Autodesk Inventor part; units mm, degrees
ref_plane "YZ Plane" through (0, 0, 0) normal (1, 0, 0) x (0, 1, 0)
ref_plane "XZ Plane" through (0, 0, 0) normal (0, 1, 0) x (-1, 0, 0)
ref_plane "XY Plane" through (0, 0, 0) normal (0, 0, 1) x (1, 0, 0)
sketch "Sketch1" plane through (0, 0, 0) normal (0, 0, 1) x (1, 0, 0)
  line L0 (-46.5, 0) -> (-46.5, -19.95)
  line L1 (-46.5, -19.95) -> (-43.5, -19.95)
  arc A0 (-6.9796, -66.5) -> (-43.5, -29.9796) centre (-45, -68) ccw
  line L2 (-43.5, -19.95) -> (-43.5, -29.9796)
  line L3 (-3, 0) -> (-3, -54.5)
  line L4 (-3, -54.5) -> (0, -54.5)
  line L5 (-20, 0) -> (-20, 3)
  line L6 (-20, 3) -> (-30, 3)
  line L7 (-30, 3) -> (-30, 0)
  line L8 (-46.5, 0) -> (-30, 0)
  line L9 (-20, 0) -> (-3, 0)
  line L10 (-3, -69.5) -> (-3, -66.5)
  line L11 (-38.5, -20.7078) -> (-38.5, -7)
  line L12 (-36.5, -5) -> (-10, -5)
  line L13 (-8, -7) -> (-8, -35.0788)
  arc A1 (-11.4568, -36.4491) -> (-36.8538, -22.6763) centre (-45, -68) ccw
  arc A2 (-38.5, -20.7078) -> (-36.8538, -22.6763) centre (-36.5, -20.7078) ccw
  arc A3 (-36.5, -5) -> (-38.5, -7) centre (-36.5, -7) ccw
  arc A4 (-8, -7) -> (-10, -5) centre (-10, -7) ccw
  arc A5 (-11.4568, -36.4491) -> (-8, -35.0788) centre (-10, -35.0788) ccw
  line L14 (-3, -66.5) -> (-6.9796, -66.5)
  line L15 (-3, -69.5) -> (0, -69.5)
  line L16 (46.5, 0) -> (46.5, -19.95)
  line L17 (46.5, -19.95) -> (43.5, -19.95)
  arc A6 (43.5, -29.9796) -> (6.9796, -66.5) centre (45, -68) ccw
  line L18 (43.5, -19.95) -> (43.5, -29.9796)
  line L19 (3, 0) -> (3, -54.5)
  line L20 (3, -54.5) -> (0, -54.5)
  line L21 (20, 0) -> (20, 3)
  line L22 (20, 3) -> (30, 3)
  line L23 (30, 3) -> (30, 0)
  line L24 (46.5, 0) -> (30, 0)
  line L25 (20, 0) -> (3, 0)
  line L26 (3, -69.5) -> (3, -66.5)
  line L27 (38.5, -20.7078) -> (38.5, -7)
  line L28 (36.5, -5) -> (10, -5)
  line L29 (8, -7) -> (8, -35.0788)
  arc A7 (36.8538, -22.6763) -> (11.4568, -36.4491) centre (45, -68) ccw
  arc A8 (36.8538, -22.6763) -> (38.5, -20.7078) centre (36.5, -20.7078) ccw
  arc A9 (38.5, -7) -> (36.5, -5) centre (36.5, -7) ccw
  arc A10 (10, -5) -> (8, -7) centre (10, -7) ccw
  arc A11 (8, -35.0788) -> (11.4568, -36.4491) centre (10, -35.0788) ccw
  line L30 (3, -66.5) -> (6.9796, -66.5)
  line L31 (3, -69.5) -> (0, -69.5)
  point P0 (0, 0)
  point P1 (-8, -40.5846)
  point P2 (-38.5, -22.411)
  point P3 (8, -40.5846)
  point P4 (38.5, -22.411)
  dimension "d1" = 46.5
  dimension "d3" = 3
  dimension "d5" = 76.1
  dimension "d7" = 45
  dimension "d10" = 10
  dimension "d24" = 10
  dimension "d25" = 20
  dimension "d29" = 3
  dimension "d32" = 8
  dimension "d33" = 5
  dimension "d36" = 17
  dimension "d37" = 16.5
  dimension "d38" = 19.95
  dimension "d39" = 5
  dimension "d40" = 2
  dimension "d45" = 8
  dimension "d49" = 69.5
  dimension "d50" = 15
extrude "Extrusion4" add sketch "Sketch1" along normal blind 3
properties part number "OpenROV 2_2 Aft Ducting Brace"
Work out the finished part from the listing and answer in its coordinate system (mm). A direction names the side the tool comes from. Round coordinates to 2 decimals unless told otherwise and drop trailing zeros. Loops run counter-clockwise (first coordinate to the right, second up) from the corner with the lowest first, then second, coordinate; pieces in that order, holes last. Notation, with made-up numbers: M 38.5,14 L 44.5,14 A25 cw 44.5,45 Z; hole C 21,-18 d7. An arc over 180 degrees is marked long. Use CSV: the item, a comma, the result in double quotes.
Q1. Section D-D, the plane z = 1.55 is taken. State how many separate pieces and enclosed holes the cut face has, then the cut area to 3 significant figures.
Determined:
separate pieces,"1"
enclosed holes,"2"
area,"2,180 mm2"
Q2. The mould has two halves that part along Y. Classify faces 5 (the flat face through (43.5, -25, 1)), 6 (the cylindrical face through (-18.377, -40.815, 1.479)), 7 (the flat face through (-23, -5, 1)): pulls with the +Y half, pulls with the -Y half, needs draft (parallel to the pull), parting line crosses it, or undercut.
Determined:
face 5,"needs draft"
face 6,"pulls with the -Y half"
face 7,"undercut"
Q3. A tool of negligible diameter and unlimited length cuts with its end or side. For faces 1 (the flat face through (5, -66.5, 1)), 2 (the flat face through (12, 0, 1)), 3 (the cylindrical face through (8.57, -5.6, 1.48)), 4 (the flat face through (-5, -66.5, 1)), from which of +Z, -Z, +X, -X, +Y, -Y can it reach the whole face along a straight path? Write none if from no direction.
Determined:
face 1,"+Z, -Z, +X, -Y"
face 2,"+Z, -Z, +Y"
face 3,"+Z, -Z"
face 4,"+Z, -Z, -X, -Y"
Q4. Section A-A, the plane y = -8 is taken. Determine the outline of the cut face in (x, z).
Determined:
outline,"M -46.5,0 L -38.5,0 L -38.5,3 L -46.5,3 Z; M -8,0 L -3,0 L -3,3 L -8,3 Z; M 3,0 L 8,0 L 8,3 L 3,3 Z; M 38.5,0 L 46.5,0 L 46.5,3 L 38.5,3 Z"
Q5. Section B-B, the plane x = 34 is taken. Determine the outline of the cut face in (y, z).
Determined:
outline,"M -31.57,0 L -23.28,0 L -23.28,3 L -31.57,3 Z; M -5,0 L 0,0 L 0,3 L -5,3 Z"
Q6. Section C-C, the plane y = -40.5 is taken. Determine the outline of the cut face in (x, z), then the cut area to 3 significant figures.
Determined:
outline,"M -18.7,0 L -3,0 L -3,3 L -18.7,3 Z; M 3,0 L 18.7,0 L 18.7,3 L 3,3 Z"
area,"94.2 mm2"
Q7. Each of these flat-tipped pins is pushed along its axis until it touches: pin 1 (1.5 mm diameter, centred on x = 6, z = 1.5, fed in from -Y); pin 2 (1.5 mm diameter, centred on y = 1.5, z = 2, fed in from +X); pin 3 (0.9 mm diameter, centred on y = -23, z = 2, fed in from +X). Where does it stop, or does it pass through?
Determined:
pin 1,"y = -66.5"
pin 2,"x = 30"
pin 3,"x = 43.5"
Q8. Consider L1, parallel to X at y = -12, z = 1.9; L2, parallel to X at y = -29, z = 1.5; L3, parallel to X at y = -2.5, z = 0.2. Determine where each line is inside the solid, lowest interval first.
Determined:
L1,"-46.5 to -38.5, -8 to -3, 3 to 8, 38.5 to 46.5"
L2,"-43.5 to -20.51, -8 to -3, 3 to 8, 20.51 to 43.5"
L3,"-46.5 to -3, 3 to 46.5"
